The drawing under review shows one solid part. Ordinate dimensions are in mm from its lowest x, y, z. A direction names the side the tool comes from. Round coordinates to 2 decimals unless told otherwise and drop trailing zeros. Write each loop counter-clockwise with the first axis right and the second up, starting at its lowest first coordinate (ties: lowest second). Pieces come first, ordered by that corner, then holes. Notation, with made-up numbers: M 47.25,11.25 L 83.25,11.25 A18 cw 83.25,45.25 Z; hole C 68,30.5 d6. An arc over 180 degrees is marked long. One line per item, written item: value. Start each with the question number.
1) Tool access review of the marked faces 5 and 6: name each direction out of +Z, -Z, +X, -X, +Y, -Y from which nothing blocks a thin tool from reaching the whole face with its end or side.
2) Mouldability with a two-part tool opening along X and no side actions: class the marked faces 1, 2, 3 and 4 as +X half, -X half, draft (parallel to the pull), parting line (faces both ways), or undercut.
3) Take a section at B-B, the plane y = 32. State how many separate pieces and enclosed holes the cut face has, and give its area (3 significant figures).
4) Take a section at D-D, the plane x = 103. Write out the cut boundary in (y, z) (1 decimal), and give its area (3 significant figures).
5) Wall thickness on probe 1 along Z at (x, y) = (70, 11.5) (1 decimal); probe 2 along Y at (x, z) = (46, 18) (1 decimal): over which ranges is each line inside the solid? List them lowest first.
6) For P1, Ø4.5, axis at x = 14.605, z = 103.505, coming from the +Y side (1 decimal); P2, Ø2, axis at x = 60, z = 90.5, coming from the +Y side (1 decimal), all flat-tipped, find the tip position at first contact; note any pin that passes through.
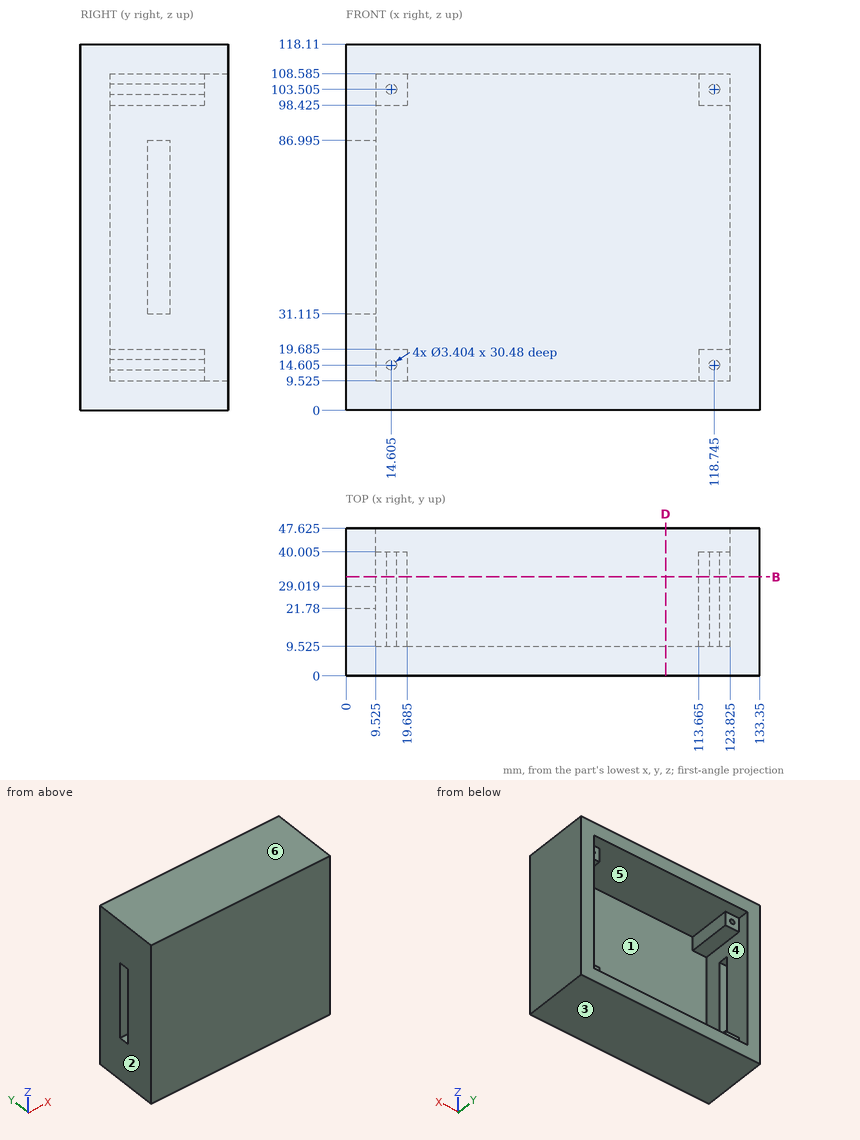
Checked values:
1. face 5: +Y
1. face 6: +Z, +X, -X, +Y, -Y
2. face 1: undercut
2. face 2: -X half
2. face 3: draft
2. face 4: undercut
3. separate pieces: 1
3. enclosed holes: 5
3. area: 4,800 mm2
4. outline: M 0,0 L 47.6,0 L 47.6,9.5 L 9.5,9.5 L 9.5,108.6 L 47.6,108.6 L 47.6,118.1 L 0,118.1 Z
4. area: 1,850 mm2
5. probe 1: z = 0 to 9.5, 108.6 to 118.1
5. probe 2: y = 0 to 9.5
6. P1: stops at y = 40
6. P2: stops at y = 9.5
